The listing builds one solid part. Answer for the finished solid, in the listing's coordinates (mm). Face numbers are marked on the shaded views. Coordinates: 2 decimals unless noted, no trailing zeros. Loops run counter-clockwise (first coordinate to the right, second up) from the corner with the lowest first, then second, coordinate; pieces in that order, holes last. Notation, with made-up numbers: M 5.25,61.5 L 43.25,61.5 A23 cw 43.25,72.5 Z; hole C -27.75,89 d11. An arc over 180 degrees is marked long. Return JSON: item names as keys, results as strings. Group by question number.
1. Section B-B (x = 8) is taken. Write down the section's boundary in (y, z), then the cut area to 3 significant figures.
2. Section A-A (z = 0) is taken. Write down the section's boundary in (x, y), then the cut area to 3 significant figures.
3. Given P1, Ø6, axis at y = 7, z = 18, coming from the -X side; P2, Ø19, axis at x = 0, z = 0, coming from the +Y side; P3, Ø2, axis at y = 7.5, z = -5.5, coming from the -X side; P4, Ø3, axis at x = 10.5, y = 10.5, coming from the +Z side, each flat-ended and moving along its own axis, determine where each tip first touches the part or whether it passes through.
4. Straight lines are drawn through the part: L1, parallel to X at y = 8.25, z = 0; L2, parallel to X at y = 7.25, z = -13; L3, parallel to Z at x = 7.5, y = 12.25. For each, find the intervals that lie inside material, in ascending order. Write a range as from..to.
5. Section D-D (x = 22) is taken. Write down the section's boundary in (y, z).
6. The mould has two halves that part along Y. Classify the marked faces 1, 2 and 3: pulls with the +Y half, pulls with the -Y half, needs draft (parallel to the pull), parting line crosses it, or undercut.
7. Section C-C (y = 14) is taken. Write down the section's boundary in (x, z).
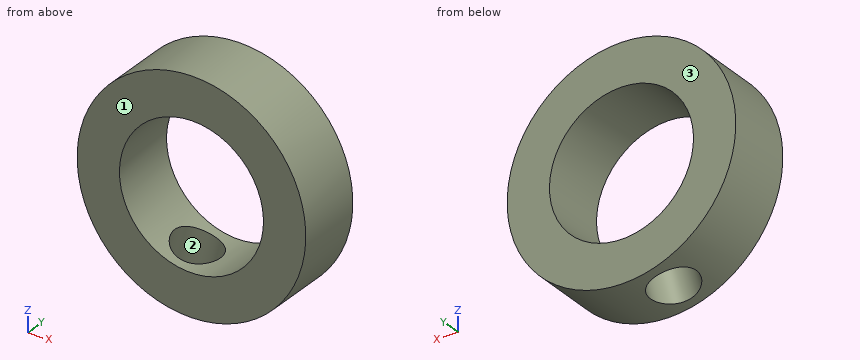
```python
from build123d import *

# Parameters (mm, degrees)
SKETCH1_R                        = 25.4
BOSS_EXTRUDE1_DEPTH              = 15
SKETCH2_R                        = 16
CUT_EXTRUDE1_DEPTH               = 15
F_10_5_10_5_DIAMETER_HOLE1_D     = 10.5
F_10_5_10_5_DIAMETER_HOLE1_DEPTH = 30
F_10_5_10_5_DIAMETER_HOLE1_TIP   = 3.15451825


with BuildPart() as part:
    # Sketch1 → Boss-Extrude1 (new body)
    with BuildSketch(Plane(origin=(0, 0, 0), x_dir=(1, 0, 0), z_dir=(0, 1, 0))):
        with Locations(Location((0, 0, 0), (0, 0, 270))):
            Circle(SKETCH1_R)
    extrude(amount=BOSS_EXTRUDE1_DEPTH)

    # Sketch2 → Cut-Extrude1 (cut)
    with BuildSketch(Plane(origin=(0, 15, 0), x_dir=(1, 0, 0), z_dir=(0, 1, 0))):
        with Locations(Location((0, 0, 0), (0, 0, 270))):
            Circle(SKETCH2_R)
    extrude(amount=-CUT_EXTRUDE1_DEPTH, mode=Mode.SUBTRACT)

    # Ø10.5 (10.5) Diameter Hole1
    with Locations(Plane(origin=(-6.456859903, 7.5, -24.565605228), x_dir=(-0.967149812109, 0, 0.254207082784), z_dir=(-0.254207082784, 0, -0.967149812109))):
        with Locations((0, 0)):
            Hole(F_10_5_10_5_DIAMETER_HOLE1_D / 2, depth=F_10_5_10_5_DIAMETER_HOLE1_DEPTH)
            with Locations((0, 0, -(F_10_5_10_5_DIAMETER_HOLE1_DEPTH + F_10_5_10_5_DIAMETER_HOLE1_TIP / 2))):  # 118° drill point
                Cone(0, F_10_5_10_5_DIAMETER_HOLE1_D / 2, F_10_5_10_5_DIAMETER_HOLE1_TIP, mode=Mode.SUBTRACT)


solid = part.part
```
Worked out:
{
 "1": {"outline": "M 0,-24.11 L 15,-24.11 L 15,-13.86 L 0,-13.86 Z; M 0,13.86 L 15,13.86 L 15,24.11 L 0,24.11 Z", "area": "308 mm^2"},
 "2": {"outline": "M -25.4,0 L -16,0 L -16,15 L -25.4,15 Z; M 16,0 L 25.4,0 L 25.4,15 L 16,15 Z", "area": "282 mm^2"},
 "3": {"P1": "x = -20.5", "P2": "through", "P3": "x = -25", "P4": "z = 23.75"},
 "4": {"L1": "-25.4..-16, 16..25.4", "L2": "-21.82..-9.33, 9.33..21.82", "L3": "-24.27..-14.13, 14.13..24.27"},
 "5": {"outline": "M 0,-12.69 L 15,-12.69 L 15,12.69 L 0,12.69 Z"},
 "6": {"face 1": "pulls with the -Y half", "face 2": "undercut", "face 3": "pulls with the +Y half"},
 "7": {"outline": "C 0,0 d50.8; hole C 0,0 d32"}
}
